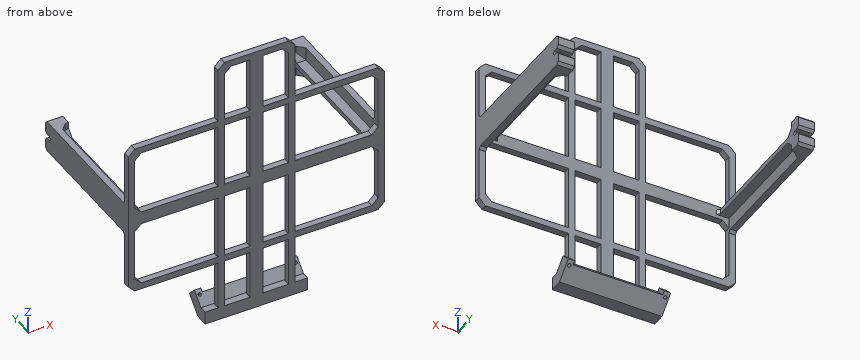
```python
from build123d import *

# Parameters (mm, degrees)
SKETCH1_W                = 200
SKETCH1_H                = 120
SKETCH1_W_2              = 190
SKETCH1_H_2              = 110
BOSS_EXTRUDE1_DEPTH      = 5
SKETCH2_W                = 5
SKETCH2_H                = 24.351612872
BOSS_EXTRUDE2_DEPTH      = 100
SKETCH3_W                = 190
SKETCH3_H                = 10
BOSS_EXTRUDE3_DEPTH      = 5
SKETCH4_W                = 12.5
SKETCH4_H                = 24.351612872
BOSS_EXTRUDE4_DEPTH      = 10
BOSS_EXTRUDE5_DEPTH      = 2
BOSS_EXTRUDE5_DEPTH_BACK = 2
SKETCH5_W                = 7.5
SKETCH5_H                = 100
CUT_EXTRUDE1_DEPTH       = 239.379948821
SKETCH7_W                = 60
SKETCH7_H                = 215.9
SKETCH7_W_2              = 50
SKETCH7_H_2              = 205.9
BOSS_EXTRUDE6_DEPTH      = 5
CHAMFER1_SIZE            = 2
SKETCH8_W                = 10
SKETCH8_H                = 205.9
BOSS_EXTRUDE7_DEPTH      = 5
CHAMFER2_SIZE            = 5
BOSS_EXTRUDE8_DEPTH      = 40
BOSS_EXTRUDE8_DEPTH_BACK = 40
SKETCH9_W                = 10
SKETCH9_H                = 5
SKETCH10_W               = 35
SKETCH10_H               = 14.142135624
SKETCH10_R               = 1.27
BOSS_EXTRUDE9_DEPTH      = 10
SKETCH12_R               = 1.27
CUT_EXTRUDE2_DEPTH       = 199.832576328


with BuildPart() as part:
    # Sketch1 → Boss-Extrude1 (new body)
    with BuildSketch(Plane(origin=(0, 0, 0), x_dir=(1, 0, 0), z_dir=(0, 1, 0))):
        Rectangle(SKETCH1_W, SKETCH1_H)
        Rectangle(SKETCH1_W_2, SKETCH1_H_2, mode=Mode.SUBTRACT)
    extrude(amount=BOSS_EXTRUDE1_DEPTH)

    # Sketch2 → Boss-Extrude2 (add)
    with BuildSketch(Plane(origin=(0, 5, 0), x_dir=(1, 0, 0), z_dir=(0, 1, 0))):
        with Locations((-97.5, 0)):
            Rectangle(SKETCH2_W, SKETCH2_H)
        with Locations((97.5, 0)):
            Rectangle(SKETCH2_W, SKETCH2_H)
    extrude(amount=BOSS_EXTRUDE2_DEPTH)

    # Sketch3 → Boss-Extrude3 (add)
    with BuildSketch(Plane.XZ):
        Rectangle(SKETCH3_W, SKETCH3_H)
    extrude(amount=-BOSS_EXTRUDE3_DEPTH)

    # Sketch4 → Boss-Extrude4 (add)
    with BuildSketch(Plane(origin=(0, 105, 0), x_dir=(1, 0, 0), z_dir=(0, 1, 0))):
        with Locations((93.75, 0)):
            Rectangle(SKETCH4_W, SKETCH4_H)
        with Locations((-93.75, 0)):
            Rectangle(SKETCH4_W, SKETCH4_H)
    extrude(amount=BOSS_EXTRUDE4_DEPTH)

    # Sketch5 → Boss-Extrude5 (add, two sides: drawn at the far end of the back side and taken through both)
    with BuildSketch(Plane.XY.offset(-BOSS_EXTRUDE5_DEPTH_BACK)):
        with Locations((-91.25, 55)):
            Rectangle(SKETCH5_W, SKETCH5_H)
        with Locations((91.25, 55)):
            Rectangle(SKETCH5_W, SKETCH5_H)
    extrude(amount=BOSS_EXTRUDE5_DEPTH + BOSS_EXTRUDE5_DEPTH_BACK)

    # Sketch6 → Cut-Extrude1 (cut, through all)
    with BuildSketch(Plane(origin=(100, 0, 0), x_dir=(0, 0, -1), z_dir=(1, 0, 0))):
        with BuildLine():
            Line((1.75, 120), (1.75, 110))
            ThreePointArc((1.75, 110), (0, 108.25), (-1.75, 110))
            Line((-1.75, 110), (-1.75, 120))
            ThreePointArc((-1.75, 120), (0, 121.75), (1.75, 120))
        make_face()
    extrude(amount=-CUT_EXTRUDE1_DEPTH, mode=Mode.SUBTRACT)

    # Sketch7 → Boss-Extrude6 (add)
    with BuildSketch(Plane(origin=(0, 5, 0), x_dir=(1, 0, 0), z_dir=(0, 1, 0))):
        Rectangle(SKETCH7_W, SKETCH7_H)
        Rectangle(SKETCH7_W_2, SKETCH7_H_2, mode=Mode.SUBTRACT)
    extrude(amount=-BOSS_EXTRUDE6_DEPTH)

    # Chamfer1
    chamfer1_edges = [part.edges().sort_by_distance(p)[0] for p in [
        (-93.75, 115, -1.75),
        (-93.75, 115, 1.75),
        (93.75, 115, 1.75),
        (93.75, 115, -1.75),
        (97.5, 5, 12.175806436),
        (87.5, 5, 0),
        (97.5, 5, -12.175806436),
        (-97.5, 5, -12.175806436),
        (-87.5, 5, 0),
        (-97.5, 5, 12.175806436),
        (-93.75, 115, 12.175806436),
        (-93.75, 115, -12.175806436),
        (93.75, 115, -12.175806436),
        (93.75, 115, 12.175806436),
    ]]
    chamfer(chamfer1_edges, length=CHAMFER1_SIZE)

    # Sketch8 → Boss-Extrude7 (add)
    with BuildSketch(Plane(origin=(0, 5, 0), x_dir=(1, 0, 0), z_dir=(0, 1, 0))):
        Rectangle(SKETCH8_W, SKETCH8_H)
    extrude(amount=-BOSS_EXTRUDE7_DEPTH)

    # Chamfer2
    chamfer2_edges = [part.edges().sort_by_distance(p)[0] for p in [
        (-95, 105, -7.087903218),
        (-91.25, 105, -2),
        (-91.25, 105, 2),
        (95, 105, 7.087903218),
        (91.25, 105, -2),
        (91.25, 105, 2),
        (-95, 2.5, 55),
        (95, 2.5, 55),
        (95, 2.5, -55),
        (-95, 2.5, -55),
        (-30, 2.5, 107.95),
        (30, 2.5, -107.95),
        (-25, 2.5, -102.95),
        (25, 2.5, 102.95),
        (-30, 2.5, -107.95),
        (30, 2.5, 107.95),
        (-25, 2.5, 102.95),
        (25, 2.5, -102.95),
        (-95, 105, 7.087903218),
        (95, 105, -7.087903218),
        (95, 2.5, 5),
        (95, 2.5, -5),
        (-95, 2.5, -5),
        (-95, 2.5, 5),
        (100, 2.5, 60),
        (-100, 2.5, 60),
        (-100, 2.5, -60),
        (100, 2.5, -60),
    ]]
    chamfer(chamfer2_edges, length=CHAMFER2_SIZE)

    # Sketch9 → Boss-Extrude8 (add, two sides: drawn at the far end of the back side and taken through both)
    with BuildSketch(Plane(origin=(0, 0, 0), x_dir=(0, 0, -1), z_dir=(1, 0, 0)).offset(-BOSS_EXTRUDE8_DEPTH_BACK)):
        Polygon((97.95, 5), (107.95, 5), (107.95, 10), (97.95, 20), align=None)
        with Locations((102.95, 2.5)):
            Rectangle(SKETCH9_W, SKETCH9_H)
    extrude(amount=BOSS_EXTRUDE8_DEPTH + BOSS_EXTRUDE8_DEPTH_BACK)

    # Sketch10 → Boss-Extrude9 (add)
    # profile 1 of 4: a face of its own
    with BuildSketch(Plane(origin=(0, 58.975, -58.975), x_dir=(1, 0, 0), z_dir=(0, 0.7071067811865489, -0.7071067811865461))):
        with Locations((-17.5, 62.190041405)):
            Rectangle(SKETCH10_W, SKETCH10_H)
    # profile 2 of 4: a face of its own
    with BuildSketch(Plane(origin=(0, 58.975, -58.975), x_dir=(1, 0, 0), z_dir=(0, 0.7071067811865489, -0.7071067811865461))):
        with Locations((17.5, 62.190041405)):
            Rectangle(SKETCH10_W, SKETCH10_H)
    # profile 3 of 4: a face of its own
    with BuildSketch(Plane(origin=(0, 58.975, -58.975), x_dir=(1, 0, 0), z_dir=(0, 0.7071067811865489, -0.7071067811865461))):
        Polygon((35, 69.261109217), (35, 55.118973593), (35, 52.261109217), (40, 52.261109217), (40, 69.261109217), align=None)
        with Locations(Location((37.425, 56.310241705, 0), (0, 0, 270))):
            Circle(SKETCH10_R, mode=Mode.SUBTRACT)
    # profile 4 of 4: a face of its own
    with BuildSketch(Plane(origin=(0, 58.975, -58.975), x_dir=(1, 0, 0), z_dir=(0, 0.7071067811865489, -0.7071067811865461))):
        Polygon((-35, 52.261109217), (-35, 55.118973593), (-35, 69.261109217), (-40, 69.261109217), (-40, 52.261109217), align=None)
        with Locations(Location((-37.425, 56.310241705, 0), (0, 0, 270))):
            Circle(SKETCH10_R, mode=Mode.SUBTRACT)
    extrude(amount=-BOSS_EXTRUDE9_DEPTH)

    # Sketch12 → Cut-Extrude2 (cut, through all)
    with BuildSketch(Plane(origin=(0, 51.903932188, -51.903932188), x_dir=(1, 0, 0), z_dir=(0, -0.7071067811865488, 0.7071067811865464))):
        with Locations(Location((37.425, -56.310241705, 0), (0, 0, 90.000000005))):
            Circle(SKETCH12_R)
        with Locations(Location((-37.425, -56.310241705, 0), (0, 0, 89.999999995))):
            Circle(SKETCH12_R)
    extrude(amount=-CUT_EXTRUDE2_DEPTH, mode=Mode.SUBTRACT)


solid = part.part
```
Input: part model. Units: mm. Frame: model coordinates. Give positions to 0.01 mm unless a question says otherwise; leave off trailing zeros. Order: outer loops, then holes, each group sorted by start corner. A loop starts at its lowest first (then second) coordinate and runs counter-clockwise, first axis right, second up. Notation, with made-up numbers: M 78,38.5 L 132,38.5 A26 cw 132,52.5 Z; hole C -33.75,-5 d2. An arc over 180 degrees is marked long. One line per question, with ' | ' between items. Start each with the question number.
1. Material intervals for probe 1 along X at (y, z) = (108.5, -6); probe 2 along Z at (x, y) = (91.5, 14); probe 3 along X at (y, z) = (60, -10), sorted ascending. Write a range as [from, to].
2. First-contact query: pin 1 Ø4 at (x, y) = (70, 1.5) entering from +Z; pin 2 Ø4 at (y, z) = (1.5, -81) entering from +X; pin 3 Ø4 at (x, y) = (48, 1.5) entering from -Z. Flat tips, straight axial feed; report the tip coordinate or a pass-through.
3. Section query B-B (y = 91). Return the cut outline in (x, z), and give its area (3 significant figures).
4. Section query A-A (z = -29.5). Return the cut outline in (x, y).
5. Section query C-C (x = 60). Return the cut outline in (y, z), and give its area (3 significant figures).
Here are the results:
1) probe 1: [-100, -87.5], [87.5, 100] | probe 2: [-2, 2] | probe 3: [-100, -95], [95, 100]
2) pin 1: z = 60 | pin 2: x = 30 | pin 3: z = -60
3) outline: M -100,-12.18 L -95,-12.18 L -95,-2 L -87.5,-2 L -87.5,2 L -95,2 L -95,12.18 L -100,12.18 Z; M 87.5,-2 L 95,-2 L 95,-12.18 L 100,-12.18 L 100,12.18 L 95,12.18 L 95,2 L 87.5,2 Z | area: 304 mm²
4) outline: M -100,0 L -95,0 L -95,5 L -100,5 Z; M -30,0 L -25,0 L -25,5 L -30,5 Z; M -5,0 L 5,0 L 5,5 L -5,5 Z; M 25,0 L 30,0 L 30,5 L 25,5 Z; M 95,0 L 100,0 L 100,5 L 95,5 Z
5) outline: M 0,-60 L 5,-60 L 5,-55 L 0,-55 Z; M 0,-5 L 5,-5 L 5,5 L 0,5 Z; M 0,55 L 5,55 L 5,60 L 0,60 Z | area: 100 mm²
